from build123d import *

# Parameters (mm, degrees)
EXTRUDE_1_DEPTH     = 37.5
CUT_EXTRUDE_1_DEPTH = 33
CUT_EXTRUDE_2_DEPTH = 33
CUT_EXTRUDE_3_DEPTH = 29
SKETCH_12_R         = 7.5
CUT_EXTRUDE_5_DEPTH = 48.765049984
CUT_EXTRUDE_6_DEPTH = 48.765049984
CUT_EXTRUDE_7_DEPTH = 48.765049984


with BuildPart() as part:
    # 草图1 → 凸台-拉伸1 (new body)
    with BuildSketch(Plane(origin=(0, 0, 0), x_dir=(1, 0, 0), z_dir=(0, 1, 0))):
        Polygon((-15, 13), (-13, 15), (13, 15), (15, 13), (15, -13), (13, -15), (-13, -15), (-15, -13), align=None)
    extrude(amount=EXTRUDE_1_DEPTH)

    # 草图2 → 切除-拉伸1 (cut)
    with BuildSketch(Plane(origin=(0, 37.5, 0), x_dir=(1, 0, 0), z_dir=(0, 1, 0))):
        Polygon((-10.5, 15), (-10.5, -15), (-13, -15), (-15, -13), (-15, 13), (-13, 15), align=None)
    extrude(amount=-CUT_EXTRUDE_1_DEPTH, mode=Mode.SUBTRACT)

    # 草图5 → 切除-拉伸2 (cut)
    with BuildSketch(Plane(origin=(0, 37.5, 0), x_dir=(1, 0, 0), z_dir=(0, 1, 0))):
        Polygon((10.5, 15), (10.5, -15), (13, -15), (15, -13), (15, 13), (13, 15), align=None)
    extrude(amount=-CUT_EXTRUDE_2_DEPTH, mode=Mode.SUBTRACT)

    # 草图6 → 切除-拉伸3 (cut)
    with BuildSketch(Plane(origin=(0, 37.5, 0), x_dir=(1, 0, 0), z_dir=(0, 1, 0))):
        Polygon((4.5, 15), (0, 15), (-4.5, 15), (-4.5, -15), (4.5, -15), align=None)
    extrude(amount=-CUT_EXTRUDE_3_DEPTH, mode=Mode.SUBTRACT)

    # 草图12 → 切除-拉伸5 (cut, through all)
    with BuildSketch(Plane(origin=(10.5, 0, 0), x_dir=(0, 0, -1), z_dir=(1, 0, 0))):
        with Locations((0, 25.5)):
            Circle(SKETCH_12_R)
    extrude(amount=-CUT_EXTRUDE_5_DEPTH, mode=Mode.SUBTRACT)

    # 草图14 → 切除-拉伸6 (cut, through all)
    with BuildSketch(Plane(origin=(10.5, 0, 0), x_dir=(0, 0, -1), z_dir=(1, 0, 0))):
        Polygon((-15, 37.5), (-13, 37.5), (-15, 35.5), align=None)
    extrude(amount=-CUT_EXTRUDE_6_DEPTH, mode=Mode.SUBTRACT)

    # 草图15 → 切除-拉伸7 (cut, through all)
    with BuildSketch(Plane(origin=(10.5, 0, 0), x_dir=(0, 0, -1), z_dir=(1, 0, 0))):
        Polygon((15, 37.5), (13, 37.5), (15, 35.5), align=None)
    extrude(amount=-CUT_EXTRUDE_7_DEPTH, mode=Mode.SUBTRACT)


solid = part.part
Design review of the part built by this model. Coordinates are the model's own, in mm. A direction names the side the tool comes from. Coordinates: 2 decimals unless noted, no trailing zeros. Order: outer loops, then holes, each group sorted by start corner. A loop starts at its lowest first (then second) coordinate and runs counter-clockwise, first axis right, second up. Notation, with made-up numbers: M 2.25,-8.75 L 27.25,-8.75 A26 cw 27.25,22.25 Z; hole C 35,60 d11. An arc over 180 degrees is marked long. Use a Markdown table: item, result.
(1) Add section B-B (z = 4.5). Give the boundary of the cut face in (x, y).
Worked answers:
| item | result |
|---|---|
| outline | M -15,0 L 15,0 L 15,4.5 L 10.5,4.5 L 10.5,19.5 L 4.5,19.5 L 4.5,8.5 L -4.5,8.5 L -4.5,19.5 L -10.5,19.5 L -10.5,4.5 L -15,4.5 Z; M -10.5,31.5 L -4.5,31.5 L -4.5,37.5 L -10.5,37.5 Z; M 4.5,31.5 L 10.5,31.5 L 10.5,37.5 L 4.5,37.5 Z |
(2) Draft analysis for pull direction Y (two halves, no side actions). For faces 1 (the flat face through (-7.5, 36.5, -14)), 2 (the cylindrical face through (7.542, 32.936, 0.976)), 3 (the flat face through (0, 0, 0)), state which applies: released by +Y, released by -Y, zero draft, split by the parting line, or undercut.
Worked answers:
| item | result |
|---|---|
| face 1 | released by +Y |
| face 2 | undercut |
| face 3 | released by -Y |
(3) Add section D-D (x = -6.5). Give the boundary of the cut face in (y, z), then the cut area to 3 significant figures.
Worked answers:
| item | result |
|---|---|
| outline | M 0,-15 L 35.5,-15 L 37.5,-13 L 37.5,13 L 35.5,15 L 0,15 Z; hole C 25.5,0 d15 |
| area | 944 mm2 |
(4) For P1, Ø8, axis at x = 11.5, y = 23.5, coming from the +Z side; P2, Ø1, axis at y = 18.5, z = 2, coming from the -X side; P3, Ø2, axis at x = 13.5, z = 7.5, coming from the +Y side; P4, Ø14.5, axis at y = 17.5, z = -5.5, coming from the +X side, all flat-tipped, find the tip position at first contact; note any pin that passes through.
Worked answers:
| item | result |
|---|---|
| P1 | stops at z = 15 |
| P2 | stops at x = -10.5 |
| P3 | stops at y = 4.5 |
| P4 | stops at x = 10.5 |
(5) Wall thickness on probe 1 along Y at (x, z) = (-7.85, 0); probe 2 along X at (y, z) = (17, 4.5); probe 3 along Y at (x, z) = (13.75, 12.5): over which ranges is each line inside the solid? List them lowest first.
Worked answers:
| item | result |
|---|---|
| probe 1 | y = 0 to 18, 33 to 37.5 |
| probe 2 | x = -10.5 to -4.5, 4.5 to 10.5 |
| probe 3 | y = 0 to 4.5 |
(6) For faces 4 (the flat face through (4.5, 17, 0)), 5 (the flat face through (10.5, 17.6, -0.2)), 6 (the flat face through (7.5, 36.5, -14)), 7 (the flat face through (6, 14, -15)), 8 (the flat face through (-13, 4.5, 0)), list the 3-axis set-ups (+Z, -Z, +X, -X, +Y, -Y) from which the entire face can be reached by the end or side of a thin tool; tool diameter is ignored.
Worked answers:
| item | result |
|---|---|
| face 4 | +Z, -Z, +Y |
| face 5 | +Z, -Z, +X, +Y |
| face 6 | -Z, +X, -X, +Y |
| face 7 | -Z, +X, -X, +Y, -Y |
| face 8 | +Z, -Z, -X, +Y |
(7) Add section C-C (y = 25.5). Give the boundary of the cut face in (x, z), then the cut area to 3 significant figures.
Worked answers:
| item | result |
|---|---|
| outline | M -10.5,-15 L -4.5,-15 L -4.5,-7.5 L -10.5,-7.5 Z; M -10.5,7.5 L -4.5,7.5 L -4.5,15 L -10.5,15 Z; M 4.5,-15 L 10.5,-15 L 10.5,-7.5 L 4.5,-7.5 Z; M 4.5,7.5 L 10.5,7.5 L 10.5,15 L 4.5,15 Z |
| area | 180 mm2 |
(8) Add section A-A (y = 10). Give the boundary of the cut face in (x, z), then the cut area to 3 significant figures.
Worked answers:
| item | result |
|---|---|
| outline | M -10.5,-15 L -4.5,-15 L -4.5,15 L -10.5,15 Z; M 4.5,-15 L 10.5,-15 L 10.5,15 L 4.5,15 Z |
| area | 360 mm2 |
